Geometry check sheet. Reference: the model listing, model coordinates, mm. Face numbers are marked on the shaded views. Give positions to 0.01 mm unless a question says otherwise; leave off trailing zeros. Loops run counter-clockwise (first coordinate to the right, second up) from the corner with the lowest first, then second, coordinate; pieces in that order, holes last. Notation, with made-up numbers: (76, 67.5) -> (110, 67.5) arc R27 ccw to (110, 89.5) -> close; hole circle Ø3 at (47.25, -3.75). An arc over 180 degrees is marked (long way). Answer in a Markdown table with one row per item. Add a question column.
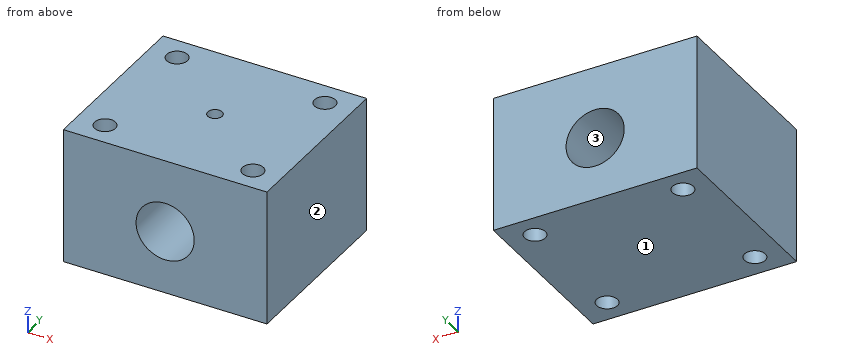
```python
from build123d import *

# Parameters (mm, degrees)
F0_W     = 42
F0_H     = 36
F0_R     = 2.15
F1_DEPTH = 28
F2_R     = 6
F3_DEPTH = 36
F4_R     = 1.5
F5_DEPTH = 5


with BuildPart() as f1:
    # F0 (on Top) → F1 (new body)
    with BuildSketch(Plane.XY):
        Rectangle(F0_W, F0_H)
        with Locations((-15.25, -13)):
            Circle(F0_R, mode=Mode.SUBTRACT)
        with Locations((15.25, -13)):
            Circle(F0_R, mode=Mode.SUBTRACT)
        with Locations((-15.25, 13)):
            Circle(F0_R, mode=Mode.SUBTRACT)
        with Locations((15.25, 13)):
            Circle(F0_R, mode=Mode.SUBTRACT)
    extrude(amount=-F1_DEPTH)

    # F2 (on face) → F3 (cut)
    with BuildSketch(Plane.XZ.offset(18)):
        with Locations((0, -15)):
            Circle(F2_R)
    extrude(amount=-F3_DEPTH, mode=Mode.SUBTRACT)

    # F4 (on face) → F5 (cut)
    with BuildSketch(Plane.XY):
        Circle(F4_R)
    extrude(amount=-F5_DEPTH, mode=Mode.SUBTRACT)


solid = f1.part
```
1. Sectioned sample at A-A (y = -13). Enter the section's corners in (x, z), plus the area to 3 significant figures.
2. Gauge pin test, flat end, axial feed: pin 1 Ø4 at (x, y) = (15.25, -13) entering from +Z. Record the tip position at first contact, or that the pin passes through.
3. Material ranges on L1, parallel to Y at x = 15.25, z = -16.25; L2, parallel to Z at x = 0, y = -1; L3, parallel to X at y = -10, z = -20, recorded low to high. Write a range as from..to.
4. Sectioned sample at C-C (x = 0). Enter the section's corners in (y, z).
5. Release check for a two-part mould opening along Z. For the marked faces 1, 2 and 3 record: released by +Z, released by -Z, zero draft, split by the parting line, or undercut.
6. Sectioned sample at D-D (x = 15.25). Enter the section's corners in (y, z).
7. Sectioned sample at B-B (z = -15). Enter the section's corners in (x, y), plus the area to 3 significant figures.
Response:
| question | item | result |
|---|---|---|
| 1 | outline | (-21, -28) -> (-17.4, -28) -> (-17.4, 0) -> (-21, 0) -> close; (-13.1, -28) -> (13.1, -28) -> (13.1, 0) -> (-13.1, 0) -> close; (17.4, -28) -> (21, -28) -> (21, 0) -> (17.4, 0) -> close; hole circle Ø12 at (0, -15) |
| 1 | area | 822 mm2 |
| 2 | pin 1 | passes through |
| 3 | L1 | y = -18..-15.15, -10.85..10.85, 15.15..18 |
| 3 | L2 | z = -28..-21, -9..-5 |
| 3 | L3 | x = -21..-3.32, 3.32..21 |
| 4 | outline | (-18, -28) -> (18, -28) -> (18, -21) -> (-18, -21) -> close; (-18, -9) -> (18, -9) -> (18, 0) -> (1.5, 0) -> (1.5, -5) -> (-1.5, -5) -> (-1.5, 0) -> (-18, 0) -> close |
| 5 | face 1 | released by -Z |
| 5 | face 2 | zero draft |
| 5 | face 3 | undercut |
| 6 | outline | (-18, -28) -> (-15.15, -28) -> (-15.15, 0) -> (-18, 0) -> close; (-10.85, -28) -> (10.85, -28) -> (10.85, 0) -> (-10.85, 0) -> close; (15.15, -28) -> (18, -28) -> (18, 0) -> (15.15, 0) -> close |
| 7 | outline | (-21, -18) -> (-6, -18) -> (-6, 18) -> (-21, 18) -> close; (6, -18) -> (21, -18) -> (21, 18) -> (6, 18) -> close; hole circle Ø4.3 at (-15.25, -13); hole circle Ø4.3 at (-15.25, 13); hole circle Ø4.3 at (15.25, -13); hole circle Ø4.3 at (15.25, 13) |
| 7 | area | 1,020 mm2 |
